Geometry check sheet. Reference: drawing and pictorial views, mm from the part's lowest x, y, z. A direction names the side the tool comes from. Give positions to 0.01 mm unless a question says otherwise; leave off trailing zeros. Order: outer loops, then holes, each group sorted by start corner. A loop starts at its lowest first (then second) coordinate and runs counter-clockwise, first axis right, second up.
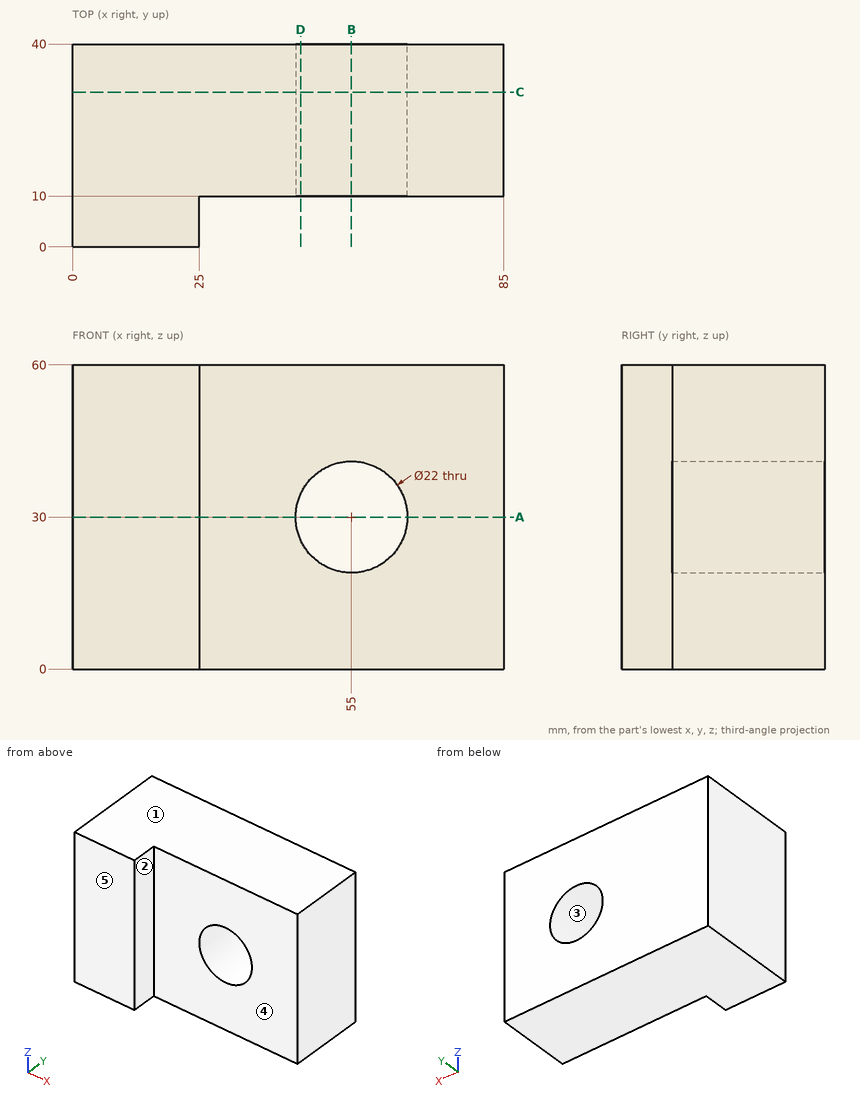
(1) Material ranges on L1, parallel to Z at x = 55, y = 27; L2, parallel to Y at x = 34, z = 23; L3, parallel to X at y = 7.5, z = 14.5, recorded low to high.
Response values:
L1: z = 0 to 19, 41 to 60
L2: y = 10 to 40
L3: x = 0 to 25
(2) Cross-section at B-B on x = 55. Enter the section's corners in (y, z), then the cut area to 3 significant figures.
Response values:
outline: (10, 0) - (40, 0) - (40, 19) - (10, 19) - close; (10, 41) - (40, 41) - (40, 60) - (10, 60) - close
area: 1,140 mm2
(3) Cross-section at C-C on y = 30.5. Enter the section's corners in (x, z), then the cut area to 3 significant figures.
Response values:
outline: (0, 0) - (85, 0) - (85, 60) - (0, 60) - close; hole circle Ø22 at (55, 30)
area: 4,720 mm2
(4) Release check for a two-part mould opening along Z. For the marked faces 1, 2 and 3 record: released by +Z, released by -Z, zero draft, split by the parting line, or undercut.
Response values:
face 1: released by +Z
face 2: zero draft
face 3: undercut
(5) Gauge pin test, flat ends, axial feed: pin 1 Ø5 at (x, y) = (25, 4.5) entering from -Z; pin 2 Ø1.5 at (y, z) = (4.5, 21) entering from +X; pin 3 Ø3 at (x, z) = (48.5, 8.5) entering from -Y; pin 4 Ø13 at (x, z) = (55, 30) entering from -Y. Record the tip position at first contact, or that the pin passes through.
Response values:
pin 1: stops at z = 0
pin 2: stops at x = 25
pin 3: stops at y = 10
pin 4: passes through
(6) Set-up check for the marked faces 4 and 5: record each of +Z, -Z, +X, -X, +Y, -Y from which the full face is reachable in a straight line by a thin tool's end or side.
Response values:
face 4: +Z, -Z, +X, -Y
face 5: +Z, -Z, +X, -X, -Y
(7) Cross-section at A-A on z = 30. Enter the section's corners in (x, y).
Response values:
outline: (0, 0) - (25, 0) - (25, 10) - (44, 10) - (44, 40) - (0, 40) - close; (66, 10) - (85, 10) - (85, 40) - (66, 40) - close
(8) Cross-section at D-D on x = 45. Enter the section's corners in (y, z).
Response values:
outline: (10, 0) - (40, 0) - (40, 25.42) - (10, 25.42) - close; (10, 34.58) - (40, 34.58) - (40, 60) - (10, 60) - close
